The figure shows three views and two pictorial views of one solid part (mm, origin at its lowest corner). Answer the questions. Coordinates: 2 decimals unless noted, no trailing zeros. Order: outer loops, then holes, each group sorted by start corner. A loop starts at its lowest first (then second) coordinate and runs counter-clockwise, first axis right, second up. Notation, with made-up numbers: M -3.5,-7 L 31.5,-7 A14 cw 31.5,6 Z; hole C -7.5,-27 d2. An arc over 180 degrees is marked long. Use a Markdown table: item, result.
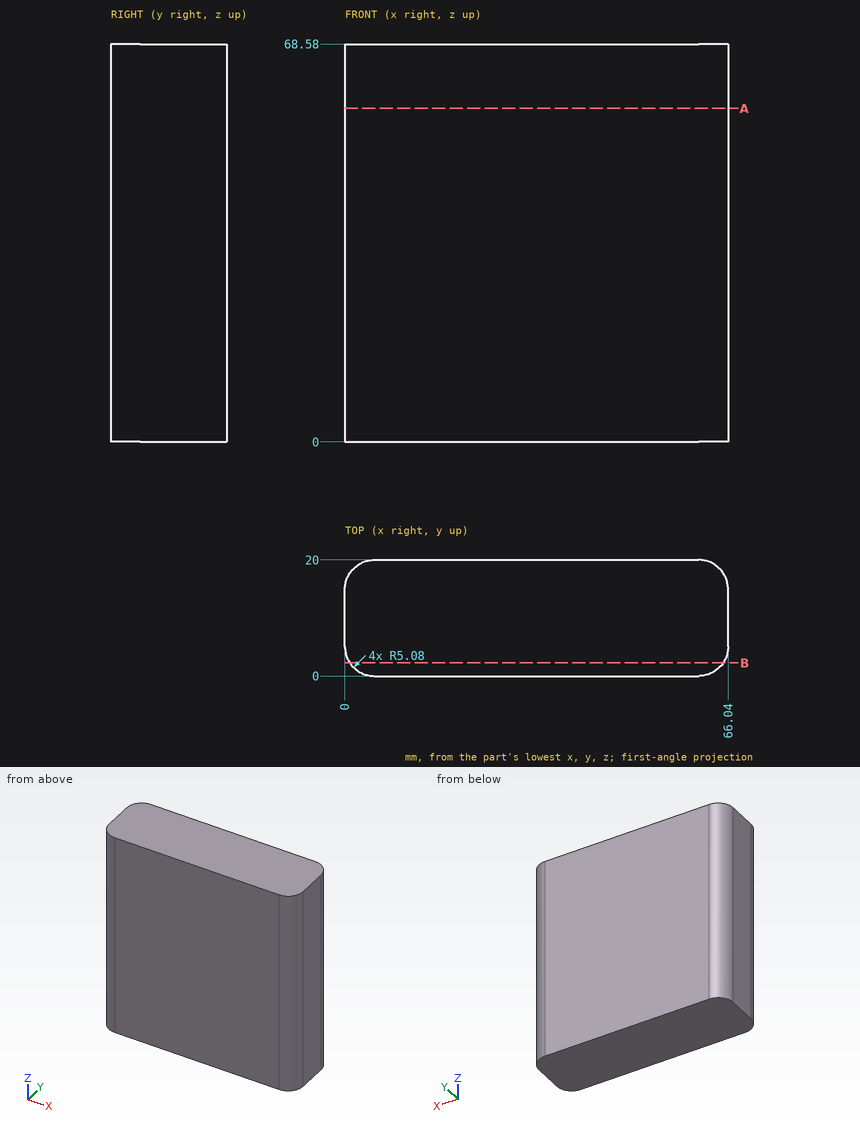
1. Section A-A on z = 57.5 is taken. Determine the outline of the cut face in (x, y), then the cut area to 3 significant figures.
Answers below:
| item | result |
|---|---|
| outline | M 0,5.08 A5.08 ccw 5.08,0 L 60.96,0 A5.08 ccw 66.04,5.08 L 66.04,14.92 A5.08 ccw 60.96,20 L 5.08,20 A5.08 ccw 0,14.92 Z |
| area | 1,300 mm² |
2. A flat-ended cylindrical pin translates along its axis: P1, Ø1, axis at y = 16.5, z = 43, coming from the -X side. Find the tip coordinate at first contact, or state that the pin passes through.
Answers below:
| item | result |
|---|---|
| P1 | x = 0.12 |
3. Find the intervals of material crossed by probe 1 along X at (y, z) = (17.25, 10.5); probe 2 along X at (y, z) = (2.25, 11.5); probe 3 along Y at (x, z) = (61.5, 29), in increasing order.
Answers below:
| item | result |
|---|---|
| probe 1 | 0.57 to 65.47 |
| probe 2 | 0.86 to 65.18 |
| probe 3 | 0.03 to 19.97 |
4. Section B-B on y = 2.25 is taken. Determine the outline of the cut face in (x, z), then the cut area to 3 significant figures.
Answers below:
| item | result |
|---|---|
| outline | M 0.86,0 L 65.18,0 L 65.18,68.58 L 0.86,68.58 Z |
| area | 4,410 mm² |
